from build123d import *

# Parameters (mm, degrees)
ESQUISSE1_W             = 12.05
ESQUISSE1_H             = 10.05
ESQUISSE1_W_2           = 10.05
ESQUISSE1_H_2           = 8.05
EXTRU_MINCE1_DEPTH      = 150
ENL_V_MAT_EXTRU_1_REACH = 152.818
ESQUISSE2_R             = 1.6
ENL_V_MAT_EXTRU_2_REACH = 152.818
ESQUISSE3_R             = 1.6


with BuildPart() as part:
    # Esquisse1 → Extru.-Mince1 (new body)
    with BuildSketch(Plane.XY):
        with Locations((6.025, 5.025)):
            Rectangle(ESQUISSE1_W, ESQUISSE1_H)
        with Locations((6.025, 5.025)):
            Rectangle(ESQUISSE1_W_2, ESQUISSE1_H_2, mode=Mode.SUBTRACT)
    extrude(amount=EXTRU_MINCE1_DEPTH)

    # Esquisse2 → Enlèv. mat.-Extru.1 (cut, up to next)
    with BuildSketch(Plane(origin=(0, 0, 0), x_dir=(-1, 0, 0), z_dir=(0, -1, 0)), mode=Mode.PRIVATE) as enl_v_mat_extru_1_sk1:
        with Locations(Location((-6.025, -80, 0), (0, 0, 90))):
            Circle(ESQUISSE2_R)
    enl_v_mat_extru_1_tool1 = extrude(enl_v_mat_extru_1_sk1.sketch, amount=-ENL_V_MAT_EXTRU_1_REACH, mode=Mode.PRIVATE) & part.part
    add(enl_v_mat_extru_1_tool1.solids().sort_by_distance((6.025, 0, 80))[0], mode=Mode.SUBTRACT)

    # Esquisse3 → Enlèv. mat.-Extru.2 (cut, up to next)
    with BuildSketch(Plane(origin=(12.05, 0, 0), x_dir=(0, 0, -1), z_dir=(1, 0, 0)), mode=Mode.PRIVATE) as enl_v_mat_extru_2_sk1:
        with Locations((-4, 5.025)):
            Circle(ESQUISSE3_R)
    enl_v_mat_extru_2_tool1 = extrude(enl_v_mat_extru_2_sk1.sketch, amount=-ENL_V_MAT_EXTRU_2_REACH, mode=Mode.PRIVATE) & part.part
    # Esquisse3 → Enlèv. mat.-Extru.2 (cut, up to next)
    with BuildSketch(Plane(origin=(12.05, 0, 0), x_dir=(0, 0, -1), z_dir=(1, 0, 0)), mode=Mode.PRIVATE) as enl_v_mat_extru_2_sk2:
        with Locations((-10, 5.025)):
            Circle(ESQUISSE3_R)
    enl_v_mat_extru_2_tool2 = extrude(enl_v_mat_extru_2_sk2.sketch, amount=-ENL_V_MAT_EXTRU_2_REACH, mode=Mode.PRIVATE) & part.part
    add(enl_v_mat_extru_2_tool1.solids().sort_by_distance((12.05, 5.025, 4))[0], mode=Mode.SUBTRACT)
    add(enl_v_mat_extru_2_tool2.solids().sort_by_distance((12.05, 5.025, 10))[0], mode=Mode.SUBTRACT)


solid = part.part
Build history of the part. All positions in model axes, mm. A direction names the side the tool comes from. Round coordinates to 2 decimals unless told otherwise and drop trailing zeros. Loops run counter-clockwise (first coordinate to the right, second up) from the corner with the lowest first, then second, coordinate; pieces in that order, holes last. Notation, with made-up numbers: (17, -19.75) -> (40, -19.75) arc R21 ccw to (40, -1.75) -> close; hole circle Ø4 at (43.5, 69). An arc over 180 degrees is marked (long way). Answer in a Markdown table with one row per item.
Item 1: Which spindle directions (+Z, -Z, +X, -X, +Y, -Y) get a long thin tool onto all of the face, cutting with end or side? Do faces 1 (the flat face through (6, 1, 74)), 2 (the cylindrical face through (6.506, 0.493, 78.474)), 3 (the cylindrical face through (11.557, 6.106, 5.179)), 4 (the flat face through (12.05, 5, 74)). Say none if no direction does.
Answers below:
| item | result |
|---|---|
| face 1 | +Z, -Z |
| face 2 | -Y |
| face 3 | +X |
| face 4 | +Z, -Z, +X, +Y, -Y |
Item 2: Mould opens along Z. For faces 5 (the cylindrical face through (11.6, 5.1, 11.6)), 6 (the flat face through (6, 9.05, 74)), 7 (the flat face through (5.9, 0.6, 150)) say: +Z half, -Z half, draft (parallel to the pull), parting line (faces both ways), or undercut.
Answers below:
| item | result |
|---|---|
| face 5 | undercut |
| face 6 | draft |
| face 7 | +Z half |
Item 3: Saw through at A-A (x = 9). Write the cut outline in (y, z).
Answers below:
| item | result |
|---|---|
| outline | (0, 0) -> (1, 0) -> (1, 150) -> (0, 150) -> close; (9.05, 0) -> (10.05, 0) -> (10.05, 150) -> (9.05, 150) -> close |
Item 4: Drill centre lines: L1, parallel to Y at x = 9, z = 86; L2, parallel to Y at x = 11.75, z = 10 (3 decimals); L3, parallel to X at y = 3, z = 76. Where is each one in solid material? Low to high. Write a range as [from, to].
Answers below:
| item | result |
|---|---|
| L1 | y = [0, 1], [9.05, 10.05] |
| L2 | y = [0, 3.425], [6.625, 10.05] |
| L3 | x = [0, 1], [11.05, 12.05] |
Item 5: Saw through at B-B (z = 55). Write the cut outline in (x, y).
Answers below:
| item | result |
|---|---|
| outline | (0, 0) -> (12.05, 0) -> (12.05, 10.05) -> (0, 10.05) -> close; hole (1, 1) -> (11.05, 1) -> (11.05, 9.05) -> (1, 9.05) -> close |
Item 6: Saw through at C-C (z = 10). Write the cut outline in (x, y) (3 decimals).
Answers below:
| item | result |
|---|---|
| outline | (0, 0) -> (12.05, 0) -> (12.05, 3.425) -> (11.05, 3.425) -> (11.05, 1) -> (1, 1) -> (1, 9.05) -> (11.05, 9.05) -> (11.05, 6.625) -> (12.05, 6.625) -> (12.05, 10.05) -> (0, 10.05) -> close |
